Here's the drawing with two shaded views (mm, measured from the low corner). I have some questions. Give positions to 0.01 mm unless a question says otherwise; leave off trailing zeros. Loops run counter-clockwise (first coordinate to the right, second up) from the corner with the lowest first, then second, coordinate; pieces in that order, holes last. Notation, with made-up numbers: M 35,5.25 L 40,5.25 A17 cw 40,29.25 Z; hole C -19.75,-20 d7. An arc over 180 degrees is marked long. Use CSV: the item, a comma, the result in double quotes.
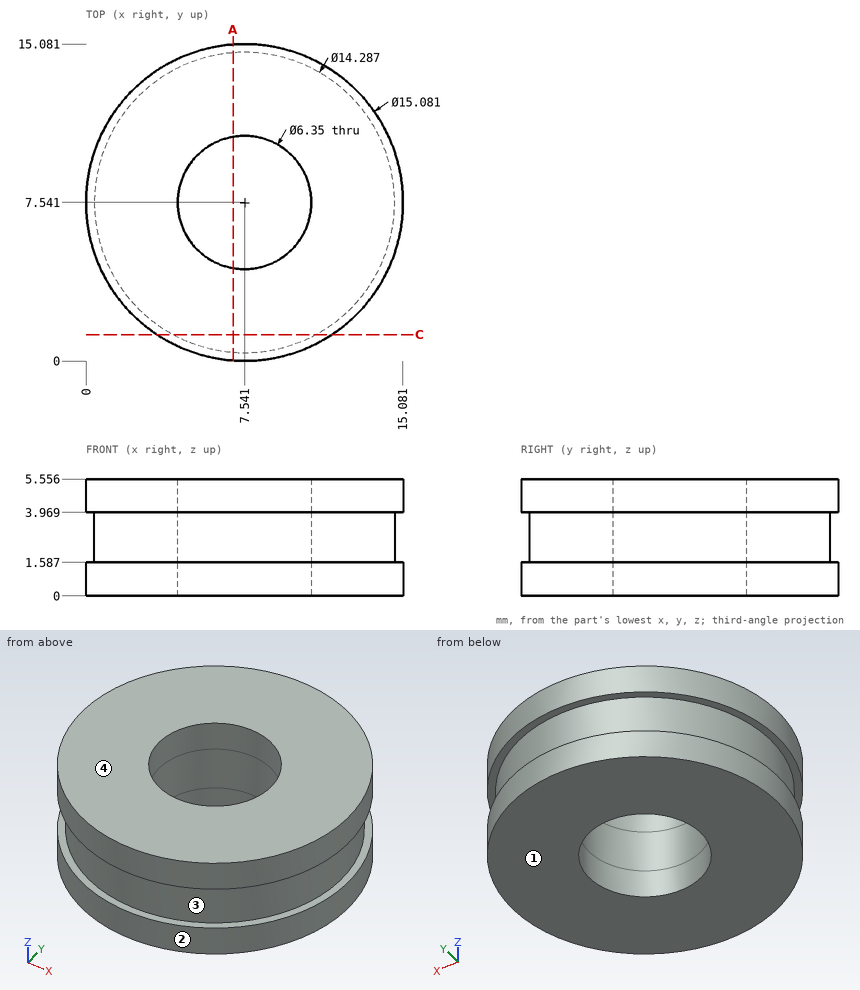
1. Please list where these lines run through material, in increasing order: line 1 (Y direction, x = 7.5, z = 2.9) (1 decimal); line 2 (Y direction, x = 5, z = 0.5) (1 decimal); line 3 (X direction, y = 8.5, z = 0.6) (1 decimal).
Outcome:
line 1,"0.4 to 4.4, 10.7 to 14.7"
line 2,"0.4 to 5.6, 9.4 to 14.6"
line 3,"0.1 to 4.5, 10.6 to 15"
2. I'm going to push flat-ended pins straight in: pin 1 Ø3 at (y, z) = (3.5, 2.5) entering from -X; pin 2 Ø1.5 at (y, z) = (8.5, 2) entering from -X; pin 3 Ø1 at (y, z) = (6, 5) entering from -X; pin 4 Ø4.5 at (x, y) = (7.5, 5.5) entering from -Z. Where does each tip first touch, or does it pass through?
Outcome:
pin 1,"x = 0.56"
pin 2,"x = 0.01"
pin 3,"x = 0.07"
pin 4,"z = 0"
3. I want a section at C-C, the plane y = 1.25. List the corners of the cut face in (x, z) for me (1 decimal).
Outcome:
outline,"M 3.4,0 L 11.7,0 L 11.7,1.6 L 10.9,1.6 L 10.9,4 L 11.7,4 L 11.7,5.6 L 3.4,5.6 L 3.4,4 L 4.2,4 L 4.2,1.6 L 3.4,1.6 Z"
4. I want a section at A-A, the plane x = 7. List the corners of the cut face in (y, z) for me.
Outcome:
outline,"M 0.02,0 L 4.41,0 L 4.41,5.56 L 0.02,5.56 L 0.02,3.97 L 0.42,3.97 L 0.42,1.59 L 0.02,1.59 Z; M 10.67,0 L 15.06,0 L 15.06,1.59 L 14.66,1.59 L 14.66,3.97 L 15.06,3.97 L 15.06,5.56 L 10.67,5.56 Z"
5. If we mould it in two halves opening along Z, with no side actions, what happens to the marked faces 1, 2, 3 and 4? For each: +Z half, -Z half, draft (parallel to the pull), parting line (faces both ways), or undercut.
Outcome:
face 1,"-Z half"
face 2,"draft"
face 3,"undercut"
face 4,"+Z half"
